Part model, mm, in its own coordinate system. A direction names the side the tool comes from. Coordinates: 2 decimals unless noted, no trailing zeros. Write each loop counter-clockwise with the first axis right and the second up, starting at its lowest first coordinate (ties: lowest second). Pieces come first, ordered by that corner, then holes. Notation, with made-up numbers: (-40, 86) -> (-17, 86) arc R20 cw to (-17, 107) -> close; hole circle Ø8 at (46, -35.5). An arc over 180 degrees is marked (long way). Write item = value, one per line.
from build123d import *

# Parameters (mm, degrees)
SKETCH2_R           = 7.9375
SKETCH2_R_2         = 3.175
BOSS_EXTRUDE1_DEPTH = 6.35


with BuildPart() as part:
    # Sketch2 → Boss-Extrude1 (new body)
    with BuildSketch(Plane(origin=(0, 69.85, 0), x_dir=(1, 0, 0), z_dir=(0, 1, 0))):
        with BuildLine():
            Line((-15.875, 6.35), (15.875, 6.35))
            Line((15.875, 6.35), (15.875, 0))
            Line((15.875, 0), (47.625, 0))
            Line((47.625, 0), (20.496649102, -231.007027591))
            ThreePointArc((20.496649102, -231.007027591), (0, -249.2375), (-20.496649102, -231.007027591))
            Line((-20.496649102, -231.007027591), (-47.625, 0))
            Line((-47.625, 0), (-15.875, 0))
            Line((-15.875, 0), (-15.875, 6.35))
        make_face()
        with Locations((0, -228.6)):
            Circle(SKETCH2_R, mode=Mode.SUBTRACT)
        with Locations((0, -214.3125)):
            Circle(SKETCH2_R_2, mode=Mode.SUBTRACT)
        with Locations((14.2875, -228.6)):
            Circle(SKETCH2_R_2, mode=Mode.SUBTRACT)
        with Locations((0, -242.8875)):
            Circle(SKETCH2_R_2, mode=Mode.SUBTRACT)
        with Locations((-14.2875, -228.6)):
            Circle(SKETCH2_R_2, mode=Mode.SUBTRACT)
    extrude(amount=BOSS_EXTRUDE1_DEPTH)


solid = part.part
Q1. Saw through at A-A on x = 0. Give the cut face in (y, z), and give its area (3 significant figures).
Model answer:
outline = (69.85, -6.35) -> (76.2, -6.35) -> (76.2, 211.14) -> (69.85, 211.14) -> close; (69.85, 217.49) -> (76.2, 217.49) -> (76.2, 220.66) -> (69.85, 220.66) -> close; (69.85, 236.54) -> (76.2, 236.54) -> (76.2, 239.71) -> (69.85, 239.71) -> close; (69.85, 246.06) -> (76.2, 246.06) -> (76.2, 249.24) -> (69.85, 249.24) -> close
area = 1,440 mm²
Q2. Pin check, flat tips, straight feed: pin 1 (3 mm diameter, centred on x = 34.5, y = 74, fed in from -Z); pin 2 (5.5 mm diameter, centred on x = 0, z = 214.31, fed in from +Y). Stop position of each tip, or through.
Model answer:
pin_1 = 0
pin_2 = through
Q3. Saw through at D-D on z = 176. Give the cut face in (x, y).
Model answer:
outline = (-26.96, 69.85) -> (26.96, 69.85) -> (26.96, 76.2) -> (-26.96, 76.2) -> close
Q4. Mould opens along X. For faces 4 (the face through (-1.72, 72.98, 236.35)), 5 (the face through (-0.41, 72.98, 239.74)), 6 (the face through (15.875, 73, -3)), 7 (the face through (-32, 73, 0)) say: released by +X, released by -X, zero draft, split by the parting line, or undercut.
Model answer:
face_4 = undercut
face_5 = undercut
face_6 = released by +X
face_7 = zero draft
Q5. Which spindle directions (+Z, -Z, +X, -X, +Y, -Y) get a long thin tool onto all of the face, cutting with end or side? Do faces 1 (the face through (32, 73, 0)), 2 (the face through (0, 73, -6.35)), 3 (the face through (-15.875, 73, -3)). Say none if no direction does.
Model answer:
face_1 = -Z, +X, +Y, -Y
face_2 = -Z, +X, -X, +Y, -Y
face_3 = -Z, -X, +Y, -Y
Q6. Saw through at C-C on z = 228.6. Give the cut face in (x, y).
Model answer:
outline = (-20.78, 69.85) -> (-17.46, 69.85) -> (-17.46, 76.2) -> (-20.78, 76.2) -> close; (-11.11, 69.85) -> (-7.94, 69.85) -> (-7.94, 76.2) -> (-11.11, 76.2) -> close; (7.94, 69.85) -> (11.11, 69.85) -> (11.11, 76.2) -> (7.94, 76.2) -> close; (17.46, 69.85) -> (20.78, 69.85) -> (20.78, 76.2) -> (17.46, 76.2) -> close
Q7. Probe line 1 (X direction, y = 72, z = 228.6); line 2 (Z direction, x = 1.5, y = 75.5); line 3 (X direction, y = 75.5, z = 49). List the from-to ranges inside material, lowest first. Write a range as from..to.
Model answer:
line_1 = -20.78..-17.46, -11.11..-7.94, 7.94..11.11, 17.46..20.78
line_2 = -6.35..211.51, 217.11..220.81, 236.39..240.09, 245.69..249.18
line_3 = -41.87..41.87
Q8. Saw through at B-B on y = 73.75. Count the separate pieces of the cut face and the enclosed holes in it, and give its area (3 significant figures).
Model answer:
separate_pieces = 1
enclosed_holes = 5
area = 16,200 mm²
